Geometry check sheet. Reference: the model listing, model coordinates, mm. Face numbers are marked on the shaded views. Coordinates: 2 decimals unless noted, no trailing zeros. Write each loop counter-clockwise with the first axis right and the second up, starting at its lowest first coordinate (ties: lowest second). Pieces come first, ordered by that corner, then holes. Notation, with made-up numbers: (31, -25.5) -> (62, -25.5) arc R21 cw to (62, -0.5) -> close; hole circle Ø4 at (59, -28.75). An arc over 180 degrees is marked (long way). Answer in a Markdown table with one row per item. Add a question column.
Q1. Gauge pin test, flat ends, axial feed: P1, Ø1.5, axis at x = 6.5, y = -5, coming from the -Z side; P2, Ø1.5, axis at x = -7.5, z = 3, coming from the -Y side; P3, Ø2, axis at x = -5, y = -3.5, coming from the -Z side. Record the tip position at first contact, or that the pin passes through.
Q2. Section check C-C, the plane y = -9.5. Record the boundary of the cut face in (x, z) (1 decimal).
Q3. Section check B-B, the plane x = 0. Record the boundary of the cut face in (y, z), and give its area (3 significant figures).
Q4. Release check for a two-part mould opening along X. For the marked faces 1 and 2 record: pulls with the +X half, pulls with the -X half, needs draft (parallel to the pull), parting line crosses it, or undercut.
Q5. Section check D-D, the plane y = -1.25. Record the boundary of the cut face in (x, z).
Q6. Section check A-A, the plane z = 0. Record the boundary of the cut face in (x, y).
Q7. Thickness scan on line 1 (Z direction, x = -2.75, y = -5); line 2 (Z direction, x = -7.5, y = 0.75); line 3 (X direction, y = 0.5, z = 2). Record the ranges inside material, lowest first.
```python
from build123d import *


with BuildPart() as part:
    # Esquisse1 → Révolution1 (revolve)
    with BuildSketch(Plane.XY, mode=Mode.PRIVATE) as r_volution1_sk:
        with BuildLine():
            Line((0, -10), (0, -9))
            ThreePointArc((0, -9), (-6.363961031, -6.363961031), (-9, 0))
            ThreePointArc((-9, 0), (-10.793209092, 1.928646174), (-12.847090142, 0.28035993))
            Line((-12.847090142, 0.28035993), (-14.5, -11))
            Line((-14.5, -11), (-13.5, -11))
            Line((-13.5, -11), (-11.857528326, 0.13624538))
            ThreePointArc((-11.857528326, 0.13624538), (-10.865455114, 0.931259132), (-10, 0))
            ThreePointArc((-10, 0), (-7.071067812, -7.071067812), (0, -10))
        make_face()
    revolve(r_volution1_sk.sketch.rotate(Axis((0, 18.017703437, 0), (0, -1, 0)), 270), axis=Axis((0, 18.017703437, 0), (0, -1, 0)))


solid = part.part
```
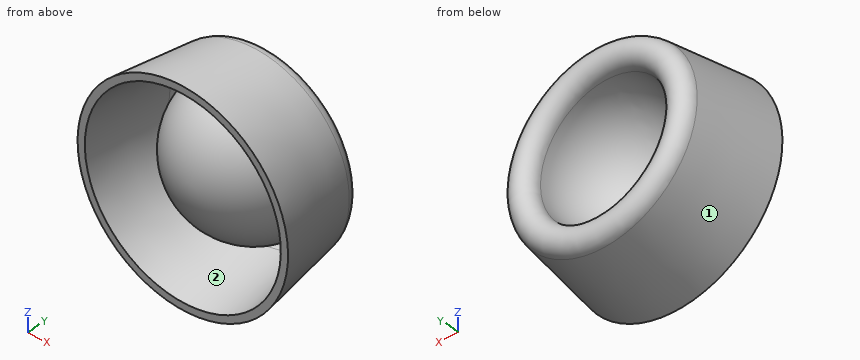
Calculated:
| question | item | result |
|---|---|---|
| 1 | P1 | stops at z = -12.37 |
| 1 | P2 | stops at y = -6.8 |
| 1 | P3 | stops at z = -12.83 |
| 2 | outline | circle Ø28.6 at (0, 0); circle Ø6.2 at (0, 0); hole circle Ø26.6 at (0, 0) |
| 3 | outline | (-11, -14.5) -> (0.28, -12.85) arc R1.93 ccw to (0, -9) arc R9 cw to (0, 9) arc R1.93 ccw to (0.28, 12.85) -> (-11, 14.5) -> (-11, 13.5) -> (0.14, 11.86) arc R0.93 cw to (0, 10) arc R10 ccw to (0, -10) arc R0.93 cw to (0.14, -11.86) -> (-11, -13.5) -> close |
| 3 | area | 61.0 mm² |
| 4 | face 1 | parting line crosses it |
| 4 | face 2 | undercut |
| 5 | outline | circle Ø26.14 at (0, 0); circle Ø19.84 at (0, 0); hole circle Ø24.12 at (0, 0); hole circle Ø17.83 at (0, 0) |
| 6 | outline | (-14.5, -11) -> (-13.5, -11) -> (-11.86, 0.14) arc R0.93 cw to (-10, 0) arc R10 ccw to (10, 0) arc R0.93 cw to (11.86, 0.14) -> (13.5, -11) -> (14.5, -11) -> (12.85, 0.28) arc R1.93 ccw to (9, 0) arc R9 cw to (-9, 0) arc R1.93 ccw to (-12.85, 0.28) -> close |
| 7 | line 1 | z = -13.34 to -12.31, -8.21 to -6.96, 6.96 to 8.21, 12.31 to 13.34 |
| 7 | line 2 | z = -10.27 to -8.7, -7.17 to -5.24, 5.24 to 7.17, 8.7 to 10.27 |
| 7 | line 3 | x = -12.64 to -11.55, -9.95 to -8.84, 8.84 to 9.95, 11.55 to 12.64 |
